Autodesk Inventor part; units mm, degrees
ref_plane "YZ Plane" through (0, 0, 0) normal (1, 0, 0) x (0, 1, 0)
ref_plane "XZ Plane" through (0, 0, 0) normal (0, 1, 0) x (-1, 0, 0)
ref_plane "XY Plane" through (0, 0, 0) normal (0, 0, 1) x (1, 0, 0)
sketch "Sketch1" plane through (0, 0, 0) normal (0, 0, 1) x (1, 0, 0)
  line L0 (1, 0) -> (209, 0)
  line L1 (178, 10) -> (32, 10)
  arc A0 (209, 0) -> (210, 1) centre (209, 1) ccw
  arc A1 (0, 1) -> (1, 0) centre (1, 1) ccw
  line L2 (27, 15) -> (27, 25)
  line L3 (22, 30) -> (1, 30)
  line L4 (1, 10) -> (5, 10)
  line L5 (5, 10) -> (5, 20)
  line L6 (5, 20) -> (1, 20)
  line L7 (0, 29) -> (0, 21)
  line L8 (0, 9) -> (0, 1)
  arc A2 (1, 30) -> (0, 29) centre (1, 29) ccw
  arc A3 (0, 21) -> (1, 20) centre (1, 21) ccw
  arc A4 (1, 10) -> (0, 9) centre (1, 9) ccw
  line L9 (183, 15) -> (183, 25)
  line L10 (188, 30) -> (209, 30)
  line L11 (209, 20) -> (205, 20)
  line L12 (205, 20) -> (205, 10)
  line L13 (205, 10) -> (209, 10)
  line L14 (210, 1) -> (210, 9)
  line L15 (210, 21) -> (210, 29)
  arc A5 (210, 29) -> (209, 30) centre (209, 29) ccw
  arc A6 (209, 20) -> (210, 21) centre (209, 21) ccw
  arc A7 (210, 9) -> (209, 10) centre (209, 9) ccw
  arc A8 (27, 25) -> (22, 30) centre (22, 25) ccw
  arc A9 (27, 15) -> (32, 10) centre (32, 15) ccw
  arc A10 (178, 10) -> (183, 15) centre (178, 15) ccw
  arc A11 (188, 30) -> (183, 25) centre (188, 25) ccw
  point P0 (0, 0)
  point P1 (183, 10)
  point P2 (27, 10)
  point P3 (27, 30)
  point P4 (0, 30)
  point P5 (210, 30)
  point P6 (183, 30)
  point P7 (210, 20)
  point P8 (210, 10)
  dimension "d0" = 10
  dimension "d2" = 1
  dimension "d8" = 27
  dimension "d9" = 10
  dimension "d11" = 5
  dimension "d12" = 1
  dimension "d13" = 27
  dimension "d14" = 5
  dimension "d15" = 10
  dimension "d16" = 10
  dimension "d17" = 30
  dimension "d18" = 1
  dimension "d19" = 30
  dimension "d20" = 210
  dimension "d21" = 5
extrude "Extrusion1" add sketch "Sketch1" along normal blind 3
properties part number "Bulkhead Brace 25100613"
Read the model definition and answer for the solid it produces. Units are mm, in the model's axes. A direction names the side the tool comes from. Coordinates: 2 decimals unless noted, no trailing zeros. Order: outer loops, then holes, each group sorted by start corner. A loop starts at its lowest first (then second) coordinate and runs counter-clockwise, first axis right, second up. Notation, with made-up numbers: (64, -15) - (98, -15) arc R26 ccw to (98, 12) - close; hole circle Ø7 at (48, 23.25). An arc over 180 degrees is marked (long way). Answer as a JSON object with one key per item and string values. Group by question number.
Item 1: Section C-C (x = 185.5) is taken. Give the vertices of the cut face in (y, z), plus the area to 3 significant figures.
Item 2: Flat-ended cylindrical pins translate along their axes: P1, Ø1.5, axis at x = 74, z = 1, coming from the +Y side; P2, Ø1.5, axis at y = 12.5, z = 2, coming from the -X side; P3, Ø0.9, axis at y = 14, z = 1, coming from the +X side. Find the tip coordinate at first contact, or state that the pin passes through.
Item 3: Section A-A (z = 0.9) is taken. Give the vertices of the cut face in (x, y), plus the area to 3 significant figures.
Item 4: The mould has two halves that part along X. Classify faces 1 (the face through (104, 9, 0)), 2 (the face through (25, 29, 1)): +X half, -X half, draft (parallel to the pull), parting line (faces both ways), or undercut.
Item 5: Section B-B (x = 122) is taken. Give the vertices of the cut face in (y, z).
Item 6: Consider probe 1 along X at (y, z) = (18.5, 2.8); probe 2 along X at (y, z) = (21, 0.85); probe 3 along Y at (x, z) = (22.5, 2.75). Determine where each line is inside the solid, lowest interval first. Write a range as from..to.
Item 7: A tool of negligible diameter and unlimited length cuts with its end or side. For faces 3 (the face through (104, 9, 3)), 4 (the face through (29, 11, 1)), from which of +Z, -Z, +X, -X, +Y, -Y can it reach the whole face along a straight path? Write none if from no direction.
Results are:
{
 "1": {"outline": "(0, 0) - (29.33, 0) - (29.33, 3) - (0, 3) - close", "area": "88.0 mm^2"},
 "2": {"P1": "stops at y = 10", "P2": "stops at x = 5", "P3": "stops at x = 205"},
 "3": {"outline": "(0, 1) arc R1 ccw to (1, 0) - (209, 0) arc R1 ccw to (210, 1) - (210, 9) arc R1 ccw to (209, 10) - (205, 10) - (205, 20) - (209, 20) arc R1 ccw to (210, 21) - (210, 29) arc R1 ccw to (209, 30) - (188, 30) arc R5 ccw to (183, 25) - (183, 15) arc R5 cw to (178, 10) - (32, 10) arc R5 cw to (27, 15) - (27, 25) arc R5 ccw to (22, 30) - (1, 30) arc R1 ccw to (0, 29) - (0, 21) arc R1 ccw to (1, 20) - (5, 20) - (5, 10) - (1, 10) arc R1 ccw to (0, 9) - close", "area": "3,080 mm^2"},
 "4": {"face 1": "draft", "face 2": "undercut"},
 "5": {"outline": "(0, 0) - (10, 0) - (10, 3) - (0, 3) - close"},
 "6": {"probe 1": "x = 5..27, 183..205", "probe 2": "x = 0..27, 183..210", "probe 3": "y = 0..29.97"},
 "7": {"face 3": "+Z, +X, -X, +Y, -Y", "face 4": "+Z, -Z, +Y"}
}
